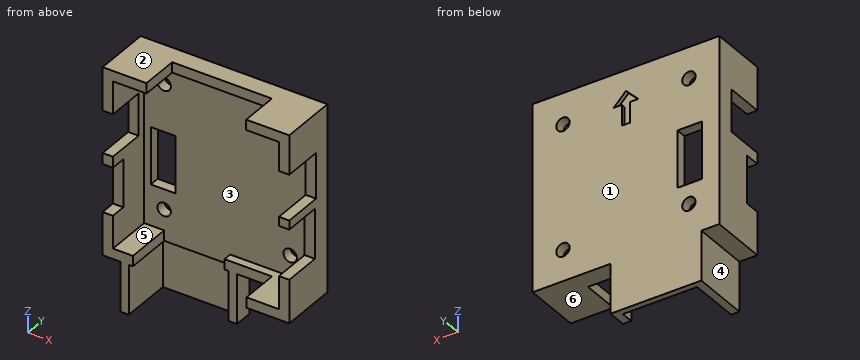
```python
from build123d import *

# Parameters (mm, degrees)
SKETCH2_W                 = 45.2
SKETCH2_H                 = 45.2
SKETCH2_W_2               = 40.2
SKETCH2_H_2               = 40.2
SKETCH2_R                 = 1.625
TOP_DEPTH                 = 2.5
SKETCH2_3_W               = 45.2
SKETCH2_3_H               = 45.2
SKETCH2_3_W_2             = 40.2
SKETCH2_3_H_2             = 40.2
SIDE_WALLS_DEPTH          = 11.3
DIRECTION_INDICATOR_DEPTH = 1
FRONT_PORTS_REACH         = 53.783
WIFI_PORT_REACH           = 36.813
SKETCH5_W                 = 6
SKETCH5_H                 = 13.8
RIGHT_PORTS_REACH         = 53.783
SKETCH6_W                 = 10.2
SKETCH6_H                 = 9.3
SKETCH6_W_2               = 11.55
SKETCH6_H_2               = 3.75
REAR_PORTS_REACH          = 53.783
SKETCH7_W                 = 16
SKETCH7_H                 = 11.3
SKETCH7_W_2               = 11.475
SKETCH7_H_2               = 9.35
LEFT_PORTS_REACH          = 53.783
SKETCH8_W                 = 12.05
SKETCH8_H                 = 9.3
BOSS_EXTRUDE3_DEPTH       = 12


with BuildPart() as part:
    # Sketch2 → Top (new body)
    # profile 1 of 2: a face of its own
    with BuildSketch(Plane(origin=(0, 0, 0), x_dir=(1, 0, 0), z_dir=(0, 1, 0))):
        Rectangle(SKETCH2_W, SKETCH2_H)
        Rectangle(SKETCH2_W_2, SKETCH2_H_2, mode=Mode.SUBTRACT)
    # profile 2 of 2: a face of its own
    with BuildSketch(Plane(origin=(0, 0, 0), x_dir=(1, 0, 0), z_dir=(0, 1, 0))):
        Rectangle(SKETCH2_W_2, SKETCH2_H_2)
        with Locations(Location((15.25, -15.075, 0), (0, 0, 270))):
            Circle(SKETCH2_R, mode=Mode.SUBTRACT)
        with Locations(Location((15.25, 15.075, 0), (0, 0, 270))):
            Circle(SKETCH2_R, mode=Mode.SUBTRACT)
        with Locations(Location((-15.25, 15.075, 0), (0, 0, 270))):
            Circle(SKETCH2_R, mode=Mode.SUBTRACT)
        with Locations(Location((-15.25, -15.075, 0), (0, 0, 270))):
            Circle(SKETCH2_R, mode=Mode.SUBTRACT)
    extrude(amount=TOP_DEPTH)

    # Sketch2<3> → Side Walls (add)
    with BuildSketch(Plane(origin=(0, 0, 0), x_dir=(1, 0, 0), z_dir=(0, 1, 0))):
        Rectangle(SKETCH2_3_W, SKETCH2_3_H)
        Rectangle(SKETCH2_3_W_2, SKETCH2_3_H_2, mode=Mode.SUBTRACT)
    extrude(amount=-SIDE_WALLS_DEPTH)

    # Sketch3 → Direction Indicator (cut)
    with BuildSketch(Plane(origin=(0, 2.5, 0), x_dir=(1, 0, 0), z_dir=(0, 1, 0))):
        Polygon((0, -17.6), (3, -14.6), (1, -14.6), (1, -9.6), (-1, -9.6), (-1, -14.6), (-3, -14.6), align=None)
    extrude(amount=-DIRECTION_INDICATOR_DEPTH, mode=Mode.SUBTRACT)

    # Sketch4 → Front Ports (cut, up to next)
    with BuildSketch(Plane.XY.offset(22.6), mode=Mode.PRIVATE) as front_ports_sk1:
        Polygon((-11.975, -2), (-0.375, -2), (0.575, -2), (12.175, -2), (12.175, -12.246111299), (0.575, -12.246111299), (-0.375, -12.246111299), (-0.375, -11.3), (-11.975, -11.3), (-11.975, -12.6), align=None)
    front_ports_tool1 = extrude(front_ports_sk1.sketch, amount=-FRONT_PORTS_REACH, mode=Mode.PRIVATE) & part.part
    add(front_ports_tool1.solids().sort_by_distance((0.391233, -6.907242, 22.6))[0], mode=Mode.SUBTRACT)

    # Sketch5 → Wifi Port (cut, up to next)
    with BuildSketch(Plane(origin=(0, 2.5, 0), x_dir=(1, 0, 0), z_dir=(0, 1, 0)), mode=Mode.PRIVATE) as wifi_port_sk1:
        with Locations((-15.475, 3.325)):
            Rectangle(SKETCH5_W, SKETCH5_H)
    wifi_port_tool1 = extrude(wifi_port_sk1.sketch, amount=-WIFI_PORT_REACH, mode=Mode.PRIVATE) & part.part
    add(wifi_port_tool1.solids().sort_by_distance((-15.475, 2.5, -3.325))[0], mode=Mode.SUBTRACT)

    # Sketch6 → Right Ports (cut, up to next)
    with BuildSketch(Plane.ZY.offset(22.6), mode=Mode.PRIVATE) as right_ports_sk1:
        with Locations((7.075, -6.65)):
            Rectangle(SKETCH6_W, SKETCH6_H)
    right_ports_tool1 = extrude(right_ports_sk1.sketch, amount=-RIGHT_PORTS_REACH, mode=Mode.PRIVATE) & part.part
    # Sketch6 → Right Ports (cut, up to next)
    with BuildSketch(Plane.ZY.offset(22.6), mode=Mode.PRIVATE) as right_ports_sk2:
        with Locations((-6.45, -9.425)):
            Rectangle(SKETCH6_W_2, SKETCH6_H_2)
    right_ports_tool2 = extrude(right_ports_sk2.sketch, amount=-RIGHT_PORTS_REACH, mode=Mode.PRIVATE) & part.part
    add(right_ports_tool1.solids().sort_by_distance((-22.6, -6.65, 7.075))[0], mode=Mode.SUBTRACT)
    add(right_ports_tool2.solids().sort_by_distance((-22.6, -9.425, -6.45))[0], mode=Mode.SUBTRACT)

    # Sketch7 → Rear Ports (cut, up to next)
    with BuildSketch(Plane(origin=(0, 0, -22.6), x_dir=(-1, 0, 0), z_dir=(0, 0, -1)), mode=Mode.PRIVATE) as rear_ports_sk1:
        with Locations((7.25, -5.65)):
            Rectangle(SKETCH7_W, SKETCH7_H)
    rear_ports_tool1 = extrude(rear_ports_sk1.sketch, amount=-REAR_PORTS_REACH, mode=Mode.PRIVATE) & part.part
    # Sketch7 → Rear Ports (cut, up to next)
    with BuildSketch(Plane(origin=(0, 0, -22.6), x_dir=(-1, 0, 0), z_dir=(0, 0, -1)), mode=Mode.PRIVATE) as rear_ports_sk2:
        with Locations((-6.4875, -6.725)):
            Rectangle(SKETCH7_W_2, SKETCH7_H_2)
    rear_ports_tool2 = extrude(rear_ports_sk2.sketch, amount=-REAR_PORTS_REACH, mode=Mode.PRIVATE) & part.part
    add(rear_ports_tool1.solids().sort_by_distance((-7.25, -5.65, -22.6))[0], mode=Mode.SUBTRACT)
    add(rear_ports_tool2.solids().sort_by_distance((6.4875, -6.725, -22.6))[0], mode=Mode.SUBTRACT)

    # Sketch8 → Left Ports (cut, up to next)
    with BuildSketch(Plane(origin=(22.6, 0, 0), x_dir=(0, 0, -1), z_dir=(1, 0, 0)), mode=Mode.PRIVATE) as left_ports_sk1:
        with Locations((6.1, -6.65)):
            Rectangle(SKETCH8_W, SKETCH8_H)
    left_ports_tool1 = extrude(left_ports_sk1.sketch, amount=-LEFT_PORTS_REACH, mode=Mode.PRIVATE) & part.part
    # Sketch8 → Left Ports (cut, up to next)
    with BuildSketch(Plane(origin=(22.6, 0, 0), x_dir=(0, 0, -1), z_dir=(1, 0, 0)), mode=Mode.PRIVATE) as left_ports_sk2:
        Polygon((-13.118203812, -9.6), (-13.118203812, -15.896164494), (-2.118203812, -15.896164494), (-2.118203812, -9.6), (-2.118203812, -1.6), (-13.118203812, -1.6), align=None)
    left_ports_tool2 = extrude(left_ports_sk2.sketch, amount=-LEFT_PORTS_REACH, mode=Mode.PRIVATE) & part.part
    add(left_ports_tool1.solids().sort_by_distance((22.6, -6.65, -6.1))[0], mode=Mode.SUBTRACT)
    add(left_ports_tool2.solids().sort_by_distance((22.6, -8.748082, 7.618204))[0], mode=Mode.SUBTRACT)

    # Sketch9 → Boss-Extrude3 (add)
    with BuildSketch(Plane(origin=(0, 0, -22.6), x_dir=(-1, 0, 0), z_dir=(0, 0, -1))):
        Polygon((-3.75, -2.05), (-1.75, -2.05), (-1.75, 1), (16.25, 1), (16.25, -11.3), (18.25, -11.3), (18.25, 2.5), (-3.75, 2.5), align=None)
    extrude(amount=BOSS_EXTRUDE3_DEPTH)


solid = part.part
```
For this review, take the finished solid that the model builds, in its own axes (mm). Face numbers are marked on the shaded views. A direction names the side the tool comes from. Coordinates: 2 decimals unless noted, no trailing zeros. Loops run counter-clockwise (first coordinate to the right, second up) from the corner with the lowest first, then second, coordinate; pieces in that order, holes last.
1. Mouldability with a two-part tool opening along Z and no side actions: class the marked faces 1, 2 and 3 as +Z half, -Z half, draft (parallel to the pull), parting line (faces both ways), or undercut.
2. For the marked faces 4, 5 and 6, list the 3-axis set-ups (+Z, -Z, +X, -X, +Y, -Y) from which the entire face can be reached by the end or side of a thin tool; tool diameter is ignored.
3. Add section C-C, the plane y = -5.25. Count the separate pieces of the cut face and the enclosed holes in it, then the cut area to 3 significant figures.
4. Insertion check: P1, Ø2, axis at x = -6.5, z = -21.5, coming from the -Y side; P2, Ø8, axis at x = -7.5, y = -4.5, coming from the -Z side; P3, Ø3, axis at x = 15.25, z = 15.075, coming from the +Y side; P4, Ø3.5, axis at x = -21.5, y = -2.5, coming from the -Z side. Each pin has a flat end and moves straight along its axis. Give the tip position at first contact, or say it passes through.
5. Add section A-A, the plane z = -7.5. Give the boundary of the cut face in (x, y) (3 decimals), then the cut area to 3 significant figures.
6. Add section B-B, the plane x = 15.25. Give the boundary of the cut face in (y, z).
7. Add section D-D, the plane z = 16. Give the boundary of the cut face in (x, y).
8. For line 1 (X direction, y = -6.75, z = -22.5) (3 decimals); line 2 (X direction, y = -2.5, z = 0.5), list the stretches that pass through material, from the lowest coordinate up.
Result:
1. face 1: draft
1. face 2: +Z half
1. face 3: undercut
2. face 4: -Z, -X, +Y, -Y
2. face 5: -Y
2. face 6: -Z, +X, +Y, -Y
3. separate pieces: 5
3. enclosed holes: 0
3. area: 239 mm2
4. P1: stops at y = 0
4. P2: stops at z = 20.1
4. P3: passes through
4. P4: stops at z = -22.6
5. outline: (-22.6, -7.55) - (-20.1, -7.55) - (-20.1, 0) - (-18.475, 0) - (-18.475, 2.5) - (-22.6, 2.5) - close; (-12.475, 0) - (20.1, 0) - (20.1, -2) - (22.6, -2) - (22.6, 2.5) - (-12.475, 2.5) - close
5. area: 122 mm2
6. outline: (-11.3, -22.6) - (2.5, -22.6) - (2.5, -16.7) - (0, -16.7) - (0, -20.1) - (-11.3, -20.1) - close; (-11.3, 20.1) - (0, 20.1) - (0, 16.7) - (2.5, 16.7) - (2.5, 22.6) - (-11.3, 22.6) - close; (0, -13.45) - (2.5, -13.45) - (2.5, 13.45) - (0, 13.45) - close
7. outline: (-22.6, -11.3) - (-20.1, -11.3) - (-20.1, 0) - (-16.59, 0) - (-16.59, 2.5) - (-22.6, 2.5) - close; (-13.91, 0) - (13.91, 0) - (13.91, 2.5) - (1.6, 2.5) - (1.6, 1.5) - (-1.6, 1.5) - (-1.6, 2.5) - (-13.91, 2.5) - close; (16.59, 0) - (20.1, 0) - (20.1, -11.3) - (22.6, -11.3) - (22.6, 2.5) - (16.59, 2.5) - close
8. line 1: x = -22.6 to -15.25, 12.225 to 22.6
8. line 2: x = -22.6 to -20.1, 20.1 to 22.6
